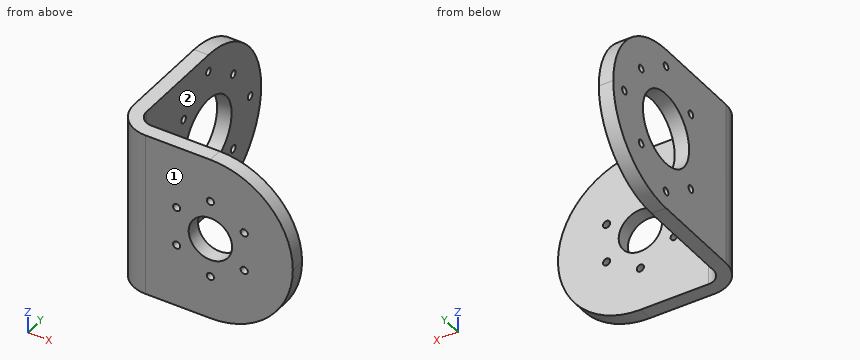
from build123d import *

# Parameters (mm, degrees)
EXTRUDE_1_DEPTH          = 57
CUT_EXTRUDE_1_DEPTH      = 57
CUT_EXTRUDE_2_DEPTH      = 57
FILLET_3_R               = 11
FILLET_4_R               = 5
SKETCH_4_R               = 12.5
SKETCH_4_R_2             = 1.25
CUT_EXTRUDE_3_DEPTH      = 57
PATTERN_CIRCULAR_1_COUNT = 4
SKETCH_5_R               = 1.25
CUT_EXTRUDE_4_DEPTH      = 57
PATTERN_CIRCULAR_2_COUNT = 3
PATTERN_CIRCULAR_2_ANGLE = 180
SKETCH_8_R               = 7.5
SKETCH_8_R_2             = 1.25
CUT_EXTRUDE_6_DEPTH      = 57
PATTERN_CIRCULAR_3_COUNT = 6


with BuildPart() as part:
    # 草图1 → 凸台-拉伸1 (new body)
    with BuildSketch(Plane.XY):
        Polygon((0, 0), (0, 72), (5, 72), (5, 5), (62, 5), (62, 0), align=None)
    extrude(amount=EXTRUDE_1_DEPTH)

    # 草图2 → 切除-拉伸1 (cut)
    with BuildSketch(Plane.ZY):
        with BuildLine():
            Line((57, 43.5), (57, 72))
            Line((57, 72), (28.5, 72))
            ThreePointArc((28.5, 72), (48.652543264, 63.652543264), (57, 43.5))
        make_face()
        with BuildLine():
            ThreePointArc((0, 43.5), (8.347456736, 63.652543264), (28.5, 72))
            Line((28.5, 72), (0, 72))
            Line((0, 72), (0, 43.5))
        make_face()
    extrude(amount=-CUT_EXTRUDE_1_DEPTH, mode=Mode.SUBTRACT)

    # 草图3 → 切除-拉伸2 (cut)
    with BuildSketch(Plane.XZ):
        with BuildLine():
            Line((62, 57), (33.5, 57))
            ThreePointArc((33.5, 57), (53.652543264, 48.652543264), (62, 28.5))
            Line((62, 28.5), (62, 57))
        make_face()
        with BuildLine():
            ThreePointArc((62, 28.5), (53.652543264, 8.347456736), (33.5, 0))
            Line((33.5, 0), (62, 0))
            Line((62, 0), (62, 28.5))
        make_face()
    extrude(amount=-CUT_EXTRUDE_2_DEPTH, mode=Mode.SUBTRACT)

    # 圆角3
    fillet_3_edges = [part.edges().sort_by_distance(p)[0] for p in [
        (0, 0, 28.5),
    ]]
    fillet(fillet_3_edges, radius=FILLET_3_R)

    # 圆角4
    fillet_4_edges = [part.edges().sort_by_distance(p)[0] for p in [
        (5, 5, 28.5),
    ]]
    fillet(fillet_4_edges, radius=FILLET_4_R)

    # 草图4 → 切除-拉伸3 (cut)
    with BuildSketch(Plane.ZY):
        with Locations((28.5, 43.5)):
            Circle(SKETCH_4_R)
        with Locations((41.935028843, 56.935028843)):
            Circle(SKETCH_4_R_2)
    cut_extrude_3 = extrude(amount=-CUT_EXTRUDE_3_DEPTH, mode=Mode.SUBTRACT)

    # 阵列(圆周)1: 切除-拉伸3 ×4 about axis
    pattern_circular_1_axis = Axis((0, 43.5, 28.5), (1, 0, 0))
    for i in range(1, PATTERN_CIRCULAR_1_COUNT):
        add(cut_extrude_3.rotate(pattern_circular_1_axis, i * 360 / PATTERN_CIRCULAR_1_COUNT), mode=Mode.SUBTRACT)

    # 草图5 → 切除-拉伸4 (cut)
    with BuildSketch(Plane.ZY):
        with Locations((51, 43.5)):
            Circle(SKETCH_5_R)
    cut_extrude_4 = extrude(amount=-CUT_EXTRUDE_4_DEPTH, mode=Mode.SUBTRACT)

    # 阵列(圆周)2: 切除-拉伸4 ×3 about axis
    pattern_circular_2_axis = Axis((0, 43.5, 28.5), (-1, 0, 0))
    for i in range(1, PATTERN_CIRCULAR_2_COUNT):
        add(cut_extrude_4.rotate(pattern_circular_2_axis, i * PATTERN_CIRCULAR_2_ANGLE / (PATTERN_CIRCULAR_2_COUNT - 1)), mode=Mode.SUBTRACT)

    # 草图8 → 切除-拉伸6 (cut)
    with BuildSketch(Plane.XZ):
        with Locations((33.5, 28.5)):
            Circle(SKETCH_8_R)
        with Locations((33.5, 15)):
            Circle(SKETCH_8_R_2)
    cut_extrude_6 = extrude(amount=-CUT_EXTRUDE_6_DEPTH, mode=Mode.SUBTRACT)

    # 阵列(圆周)3: 切除-拉伸6 ×6 about axis
    pattern_circular_3_axis = Axis((33.5, 0, 28.5), (0, 1, 0))
    for i in range(1, PATTERN_CIRCULAR_3_COUNT):
        add(cut_extrude_6.rotate(pattern_circular_3_axis, i * 360 / PATTERN_CIRCULAR_3_COUNT), mode=Mode.SUBTRACT)


solid = part.part
Here's how the part is built. I have some questions about the finished solid (model axes, mm). Face numbers are marked on the shaded views. A direction names the side the tool comes from. Give positions to 0.01 mm unless a question says otherwise; leave off trailing zeros. Write each loop counter-clockwise with the first axis right and the second up, starting at its lowest first coordinate (ties: lowest second). Pieces come first, ordered by that corner, then holes. Notation, with made-up numbers: (68, -8.5) -> (87, -8.5) arc R29 cw to (87, 21.5) -> close; hole circle Ø5 at (-21, 67). An arc over 180 degrees is marked (long way). Use one line per item in the form item = value. Start each with the question number.
1. If I drill on L1, parallel to Z at x = 33.5, y = 2.35; L2, parallel to X at y = 2.35, z = 21.75; L3, parallel to Y at x = 43, z = 2.5, over which ranges is the centre line in solid material (lowest first)?
2. On a 3-axis mill with a long thin cutter (end or side, diameter ignored), from which of +Z, -Z, +X, -X, +Y, -Y can I reach the whole of each face in a straight line? I mean the marked faces 1 and 2. Say none if no direction works.
3. Will these pins go through, and if not, where does the flat tip stop? pin 1 Ø3 at (y, z) = (56.94, 15.06) entering from -X; pin 2 Ø17 at (x, z) = (33.5, 28.5) entering from +Y; pin 3 Ø5 at (y, z) = (23, 48.5) entering from +X.
4. Imagine slicing it at C-C on z = 44.5. List the corners of the cut face in (x, y) for me, plus the area to 3 significant figures.
5. Imagine slicing it at B-B on z = 6. List the corners of the cut face in (x, y) for me, plus the area to 3 significant figures.
6. Imagine slicing it at A-A on y = 66. List the corners of the cut face in (x, z) for me, plus the area to 3 significant figures.
7. Imagine slicing it at D-D on y = 27. List the corners of the cut face in (x, z) for me, plus the area to 3 significant figures.
Entries:
q1.L1 = 0 to 13.75, 16.25 to 21, 36 to 40.75, 43.25 to 57
q1.L2 = 4.2 to 20.56, 23.06 to 30.23, 36.77 to 43.94, 46.44 to 61.19
q1.L3 = 0 to 5
q2.face_1 = +Z, -Z, +X, -X, -Y
q2.face_2 = +Z, -Z, +X, +Y
q3.pin_1 = 0
q3.pin_2 = 5
q3.pin_3 = 5
q4.outline = (0, 11) arc R11 ccw to (11, 0) -> (57.08, 0) -> (57.08, 5) -> (10, 5) arc R5 cw to (5, 10) -> (5, 67.08) -> (0, 67.08) -> close
q4.area = 575 mm²
q5.outline = (0, 11) arc R11 ccw to (11, 0) -> (50.99, 0) -> (50.99, 5) -> (10, 5) arc R5 cw to (5, 10) -> (5, 42.25) -> (0, 42.25) -> close; (0, 44.75) -> (5, 44.75) -> (5, 60.99) -> (0, 60.99) -> close
q5.area = 502 mm²
q6.outline = (0, 11.01) -> (5, 11.01) -> (5, 27.25) -> (0, 27.25) -> close; (0, 29.75) -> (5, 29.75) -> (5, 45.99) -> (0, 45.99) -> close
q6.area = 162 mm²
q7.outline = (0, 0) -> (5, 0) -> (5, 57) -> (0, 57) -> close
q7.area = 285 mm²
